CAD build for the part. Positions are in the model's coordinates, mm. Face numbers are marked on the shaded views. A direction names the side the tool comes from. Round coordinates to 2 decimals unless told otherwise and drop trailing zeros. Order: outer loops, then holes, each group sorted by start corner. A loop starts at its lowest first (then second) coordinate and runs counter-clockwise, first axis right, second up. Notation, with made-up numbers: (75, 22.5) -> (117, 22.5) arc R15 cw to (117, 36.5) -> close; hole circle Ø5 at (33, 68). An arc over 180 degrees is marked (long way). Return JSON: item names as keys, results as strings. Group by question number.
Q1. Mould opens along Z. For the marked faces 1, 2, 3 and 4 say: +Z half, -Z half, draft (parallel to the pull), parting line (faces both ways), or undercut.
Q2. Which spindle directions (+Z, -Z, +X, -X, +Y, -Y) get a long thin tool onto all of the face, cutting with end or side? Do the marked faces 5, 6 and 7. Say none if no direction does.
Q3. Cut at C-C (z = 18). Write the cut outline in (x, y) (3 decimals).
Q4. Probe line 1 along Z through (x, y) = (9, 2.75); line 2 along Z through (x, y) = (2.75, -3.75); line 3 along X through (y, z) = (0.25, 2.5). List the from-to ranges inside material, lowest first.
Q5. Flat gauge pins, fed straight in: pin 1 (0.5 mm diameter, centred on y = -0.5, z = 33, fed in from +X); pin 2 (3.5 mm diameter, centred on x = 2, y = 1.5, fed in from -Z); pin 3 (1 mm diameter, centred on x = -7.5, z = 17.5, fed in from -Y). Where does each tip first touch, or does it go through?
Q6. Cut at B-B (x = 9). Write the cut outline in (y, z), then the cut area to 3 significant figures.
Q7. Cut at D-D (x = -5.5). Write the cut outline in (y, z) (3 decimals), then the cut area to 3 significant figures.
Q8. Cut at A-A (z = 2.5). Write the cut outline in (x, y) (3 decimals), then the cut area to 3 significant figures.
from build123d import *

# Parameters (mm, degrees)
SKETCH1_W               = 20
SKETCH1_H               = 11.5
BOSS_EXTRUDE1_DEPTH     = 5
SKETCH2_W               = 5
SKETCH2_H               = 11.5
BOSS_EXTRUDE2_DEPTH     = 25
SKETCH3_W               = 18
SKETCH3_H               = 11.75
BOSS_EXTRUDE3_DEPTH     = 5
CUT_EXTRUDE1_DEPTH      = 5
CUT_EXTRUDE2_DEPTH      = 33.186953879
CUT_EXTRUDE2_DEPTH_BACK = 33.186953879
SKETCH5_R               = 2
FILLET1_R               = 9
FILLET7_R               = 5
FILLET8_R               = 1
FILLET9_R               = 2
CUT_EXTRUDE4_DEPTH      = 39.173943993
CUT_EXTRUDE4_DEPTH_BACK = 39.173943993
SKETCH10_R              = 1.5
SKETCH10_4_R            = 3.5
SKETCH10_4_R_2          = 1.5
BOSS_EXTRUDE7_DEPTH     = 11.5
FILLET13_R              = 1
FILLET16_R              = 5
FILLET17_R              = 3


with BuildPart() as part:
    # Sketch1 → Boss-Extrude1 (new body)
    with BuildSketch(Plane.XY):
        Rectangle(SKETCH1_W, SKETCH1_H)
    extrude(amount=BOSS_EXTRUDE1_DEPTH)

    # Sketch2 → Boss-Extrude2 (add)
    with BuildSketch(Plane.XY.offset(5)):
        with Locations((-7.5, 0)):
            Rectangle(SKETCH2_W, SKETCH2_H)
    extrude(amount=BOSS_EXTRUDE2_DEPTH)

    # Sketch3 → Boss-Extrude3 (add)
    with BuildSketch(Plane.XY.offset(30)):
        with Locations((-1, -0.125)):
            Rectangle(SKETCH3_W, SKETCH3_H)
    extrude(amount=BOSS_EXTRUDE3_DEPTH)

    # Sketch4 → Cut-Extrude1 (cut)
    with BuildSketch(Plane.ZY.offset(10)):
        with BuildLine():
            Line((15, 2.875), (25, 2.875))
            ThreePointArc((25, 2.875), (28, -0.125), (25, -3.125))
            Line((25, -3.125), (15, -3.125))
            ThreePointArc((15, -3.125), (12, -0.125), (15, 2.875))
        make_face()
    extrude(amount=-CUT_EXTRUDE1_DEPTH, mode=Mode.SUBTRACT)

    # Sketch5 → Cut-Extrude2 (cut, two sides: drawn at the far end of the back side and taken through both)
    with BuildSketch(Plane(origin=(0, 0, 30), x_dir=(-1, 0, 0), z_dir=(0, 0, -1)).offset(-CUT_EXTRUDE2_DEPTH_BACK)):
        with Locations((-2, -0.125)):
            Circle(SKETCH5_R)
    extrude(amount=CUT_EXTRUDE2_DEPTH + CUT_EXTRUDE2_DEPTH_BACK, mode=Mode.SUBTRACT)

    # Fillet1
    fillet1_edges = [part.edges().sort_by_distance(p)[0] for p in [
        (-10, 0, 0),
    ]]
    fillet(fillet1_edges, radius=FILLET1_R)

    # Fillet7
    fillet7_edges = [part.edges().sort_by_distance(p)[0] for p in [
        (8, -6, 32.5),
        (8, 5.75, 32.5),
    ]]
    fillet(fillet7_edges, radius=FILLET7_R)

    # Fillet8
    fillet8_edges = [part.edges().sort_by_distance(p)[0] for p in [
        (-10, -0.125, 12),
        (-10, -3.125, 20),
        (-10, -0.125, 28),
        (-10, 2.875, 20),
    ]]
    fillet(fillet8_edges, radius=FILLET8_R)

    # Fillet9
    fillet9_edges = [part.edges().sort_by_distance(p)[0] for p in [
        (-5, -0.125, 12),
        (-5, 2.875, 20),
        (-5, -0.125, 28),
        (-5, -3.125, 20),
    ]]
    fillet(fillet9_edges, radius=FILLET9_R - 0.0001)  # a hair under: the kernel refuses the full size

    # Sketch10 → Cut-Extrude4 (cut, two sides: drawn at the far end of the back side and taken through both)
    with BuildSketch(Plane.XZ.offset(5.75).offset(-CUT_EXTRUDE4_DEPTH_BACK)):
        with Locations((9, 2.5)):
            Circle(SKETCH10_R)
    extrude(amount=CUT_EXTRUDE4_DEPTH + CUT_EXTRUDE4_DEPTH_BACK, mode=Mode.SUBTRACT)

    # Sketch10<4> → Boss-Extrude7 (add)
    with BuildSketch(Plane.XZ.offset(5.75)):
        with Locations((9, 2.5)):
            Circle(SKETCH10_4_R)
        with Locations(Location((9, 2.5, 0), (0, 0, 270))):
            Circle(SKETCH10_4_R_2, mode=Mode.SUBTRACT)
    extrude(amount=-BOSS_EXTRUDE7_DEPTH)

    # Fillet13
    fillet13_edges = [part.edges().sort_by_distance(p)[0] for p in [
        (6.550510257, 0, 0),
        (6.550510257, 0, 5),
    ]]
    fillet(fillet13_edges, radius=FILLET13_R)

    # Fillet16
    fillet16_edges = [part.edges().sort_by_distance(p)[0] for p in [
        (-5, 0, 5),
    ]]
    fillet(fillet16_edges, radius=FILLET16_R - 0.0001)  # a hair under: the kernel refuses the full size

    # Fillet17
    fillet17_edges = [part.edges().sort_by_distance(p)[0] for p in [
        (-10, -0.125, 35),
    ]]
    fillet(fillet17_edges, radius=FILLET17_R)


solid = part.part
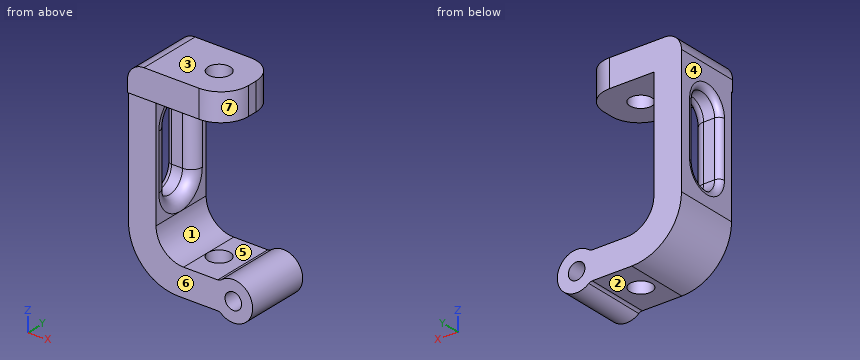
Solution:
{
 "1": {"face 1": "undercut", "face 2": "-Z half", "face 3": "+Z half", "face 4": "draft"},
 "2": {"face 5": "+Y, -Y", "face 6": "-Z, +X, -X, -Y", "face 7": "+Z, +X, -Y"},
 "3": {"outline": "(-10, -5.75) -> (-5, -5.75) -> (-5, -5.125) arc R2 ccw to (-7, -3.125) -> (-9, -3.125) arc R1 ccw to (-10, -4.125) -> close; (-10, 3.875) arc R1 ccw to (-9, 2.875) -> (-7, 2.875) arc R2 ccw to (-5, 4.875) -> (-5, 5.75) -> (-10, 5.75) -> close"},
 "4": {"line 1": "z = -1 to 1, 4 to 6", "line 2": "z = 0 to 5, 30 to 35", "line 3": "x = -7.22 to 0.04, 3.96 to 7.5, 10.5 to 12.5"},
 "5": {"pin 1": "stops at x = 8", "pin 2": "stops at z = 0", "pin 3": "stops at y = -5.75"},
 "6": {"outline": "(-5.75, -1) -> (5.75, -1) -> (5.75, 1) -> (-5.75, 1) -> close; (-5.75, 4) -> (5.75, 4) -> (5.75, 6) -> (-5.75, 6) -> close", "area": "46.0 mm²"},
 "7": {"outline": "(-6, 30) -> (-5.75, 30) -> (-5.75, 1.206) -> (5.75, 1.206) -> (5.75, 35) -> (-6, 35) -> close; hole (-3.802, 15) arc R3.677 ccw to (3.552, 15) -> (3.552, 25) arc R3.677 ccw to (-3.802, 25) -> close", "area": "274 mm²"},
 "8": {"outline": "(-7.225, -5.75) -> (7.5, -5.75) -> (7.5, 5.75) -> (-7.225, 5.75) -> close; (10.5, -5.75) -> (12.5, -5.75) -> (12.5, 5.75) -> (10.5, 5.75) -> close; hole circle Ø4 at (2, -0.125)", "area": "180 mm²"}
}
